The figure shows three views and two pictorial views of one solid part (mm, origin at its lowest corner). Answer the questions. A direction names the side the tool comes from. Coordinates: 2 decimals unless noted, no trailing zeros. Loops run counter-clockwise (first coordinate to the right, second up) from the corner with the lowest first, then second, coordinate; pieces in that order, holes last. Notation, with made-up numbers: (-10.5, 86) -> (-1.5, 86) arc R31 ccw to (-1.5, 110) -> close; hole circle Ø1 at (15, 51.25). An arc over 180 degrees is marked (long way). Answer in a Markdown table with one row per item.
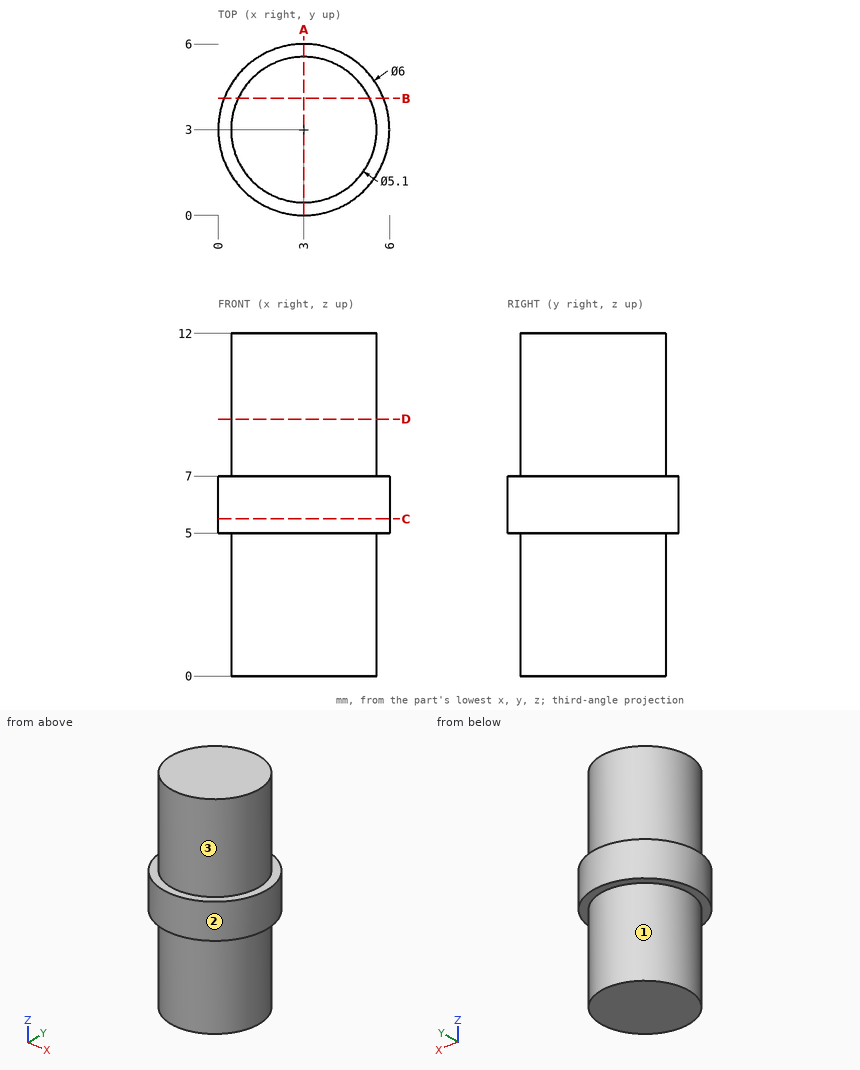
Item 1: Flat-ended cylindrical pins translate along their axes: pin 1 Ø2 at (x, z) = (2, 2) entering from +Y; pin 2 Ø1.5 at (x, z) = (5.5, 8.5) entering from -Y; pin 3 Ø1 at (y, z) = (3.5, 9) entering from +X. Find the tip coordinate at first contact, or state that the pin passes through.
Findings below:
| item | result |
|---|---|
| pin 1 | stops at y = 5.55 |
| pin 2 | stops at y = 1.15 |
| pin 3 | stops at x = 5.55 |
Item 2: A tool of negligible diameter and unlimited length cuts with its end or side. For the marked faces 1, 2 and 3, from which of +Z, -Z, +X, -X, +Y, -Y can it reach the whole face along a straight path? Write none if from no direction.
Findings below:
| item | result |
|---|---|
| face 1 | -Z |
| face 2 | +Z, -Z |
| face 3 | +Z |
Item 3: A cutting plane is placed at C-C, the plane z = 5.5. Determine the outline of the cut face in (x, y), plus the area to 3 significant figures.
Findings below:
| item | result |
|---|---|
| outline | circle Ø6 at (3, 3) |
| area | 28.3 mm2 |
Item 4: A cutting plane is placed at D-D, the plane z = 9. Determine the outline of the cut face in (x, y), plus the area to 3 significant figures.
Findings below:
| item | result |
|---|---|
| outline | circle Ø5.1 at (3, 3) |
| area | 20.4 mm2 |
Item 5: A cutting plane is placed at A-A, the plane x = 3. Determine the outline of the cut face in (y, z).
Findings below:
| item | result |
|---|---|
| outline | (0, 5) -> (0.45, 5) -> (0.45, 0) -> (5.55, 0) -> (5.55, 5) -> (6, 5) -> (6, 7) -> (5.55, 7) -> (5.55, 12) -> (0.45, 12) -> (0.45, 7) -> (0, 7) -> close |
Item 6: Find the intervals of material crossed by probe 1 along Z at (x, y) = (5.7, 3.9); probe 2 along Y at (x, z) = (4.55, 6); probe 3 along X at (y, z) = (5.15, 10.25), in increasing order.
Findings below:
| item | result |
|---|---|
| probe 1 | z = 5 to 7 |
| probe 2 | y = 0.43 to 5.57 |
| probe 3 | x = 1.63 to 4.37 |
Item 7: A cutting plane is placed at B-B, the plane y = 4.1. Determine the outline of the cut face in (x, z).
Findings below:
| item | result |
|---|---|
| outline | (0.21, 5) -> (0.7, 5) -> (0.7, 0) -> (5.3, 0) -> (5.3, 5) -> (5.79, 5) -> (5.79, 7) -> (5.3, 7) -> (5.3, 12) -> (0.7, 12) -> (0.7, 7) -> (0.21, 7) -> close |
